Design review of the part built by this model. Coordinates are the model's own, in mm. Coordinates: 2 decimals unless noted, no trailing zeros. Order: outer loops, then holes, each group sorted by start corner. A loop starts at its lowest first (then second) coordinate and runs counter-clockwise, first axis right, second up.
from build123d import *

# Parameters (mm, degrees)
SWEEP1_PROFILE_R    = 2
BOSS_EXTRUDE1_DEPTH = 5
SKETCH10_R          = 1.75
CUT_EXTRUDE1_DEPTH  = 200
SKETCH35_R          = 1.5
CUT_EXTRUDE3_DEPTH  = 10


with BuildPart() as part:
    # Sweep1: sweep along a path in Sketch2
    with BuildLine(Plane(origin=(0, 0, 0), x_dir=(1, 0, 0), z_dir=(0, 1, 0))) as sweep1_path:
        Line((-100, 0), (100, 0))
    # Sweep1 profile (on start of the path) → Sweep1 (sweep)
    with BuildSketch(Plane(origin=(-100, 0, 0), x_dir=(0, 0, 1), z_dir=(1, 0, 0))):
        Circle(SWEEP1_PROFILE_R)
    sweep(path=sweep1_path.line)

    # Sketch9 → Boss-Extrude1 (add)
    with BuildSketch(Plane.ZY.offset(100)):
        Polygon((1.98826653, -1.174789146), (2.01153051, 1.134494752), (0.023263979, 2.309283898), (-1.98826653, 1.174789146), (-2.01153051, -1.134494752), (-0.023263979, -2.309283898), align=None)
    extrude(amount=BOSS_EXTRUDE1_DEPTH)

    # Sketch10 → Cut-Extrude1 (cut)
    with BuildSketch(Plane(origin=(100, 0, 0), x_dir=(0, 0, -1), z_dir=(1, 0, 0))):
        Circle(SKETCH10_R)
    extrude(amount=-CUT_EXTRUDE1_DEPTH, mode=Mode.SUBTRACT)

    # Sketch35 → Cut-Extrude3 (cut)
    with BuildSketch(Plane.XY.offset(2)):
        with Locations((65, 0)):
            Circle(SKETCH35_R)
        with Locations((-65, 0)):
            Circle(SKETCH35_R)
    extrude(amount=-CUT_EXTRUDE3_DEPTH, mode=Mode.SUBTRACT)


solid = part.part
1. Add section A-A (x = 29.5). Give the boundary of the cut face in (y, z), and give its area (3 significant figures).
2. Insertion check: pin 1 (1.5 mm diameter, centred on x = 67, z = 0.5, fed in from -Y); pin 2 (1 mm diameter, centred on x = -45, y = 1.5, fed in from +Z). Each pin has a flat end and moves straight along its axis. Give the tip position at first contact, or say it passes through.
3. Mouldability with a two-part tool opening along Z and no side actions: class faces 1 (the flat face through (-105, 0, 0)), 2 (the cylindrical face through (1.4, -1.71, 0.38)), 3 (the cylindrical face through (1.4, 0.766, 1.847)), 4 (the flat face through (-100, 0, 0)) as pulls with the +Z half, pulls with the -Z half, needs draft (parallel to the pull), parting line crosses it, or undercut.
4. To check wall thickness, follow line 1 (Y direction, x = -78, z = 0.3); line 2 (Z direction, x = -73, y = 0.1); line 3 (X direction, y = 0.6, z = 1.2). State the ranges of each line that lie inside material, in increasing order.
Solution:
1. outline: circle Ø4 at (0, 0); hole circle Ø3.5 at (0, 0)
1. area: 2.95 mm2
2. pin 1: stops at y = -2
2. pin 2: stops at z = 1.73
3. face 1: needs draft
3. face 2: undercut
3. face 3: parting line crosses it
3. face 4: undercut
4. line 1: y = -1.98 to -1.72, 1.72 to 1.98
4. line 2: z = -2 to -1.75, 1.75 to 2
4. line 3: x = -105 to -100
